Check sheet for the modelled part. Datum: model origin and axes. Units: mm. A direction names the side the tool comes from. Round coordinates to 2 decimals unless told otherwise and drop trailing zeros. Write each loop counter-clockwise with the first axis right and the second up, starting at its lowest first coordinate (ties: lowest second). Pieces come first, ordered by that corner, then holes.
Item 1: Cross-section at A-A on y = 0. Enter the section's corners in (x, z).
Item 2: Cross-section at C-C on x = 3.25. Enter the section's corners in (y, z).
Item 3: Cross-section at D-D on z = 1. Count the separate pieces of the cut face and the enclosed holes in it, plus the area to 3 significant figures.
Item 4: Cross-section at B-B on x = 1. Enter the section's corners in (y, z), plus the area to 3 significant figures.
Item 5: Go/stop test with flat-tipped pins: pin 1 Ø1.5 at (y, z) = (4.5, 5) entering from -X; pin 2 Ø1.4 at (x, y) = (-0.89, 3.33) entering from -Z; pin 3 Ø3 at (x, z) = (-3.5, 4) entering from +Y; pin 4 Ø3 at (y, z) = (4.5, 4) entering from +X. Record where each tip stops, or that it passes through.
Item 6: Material ranges on line 1 (Y direction, x = 1.25, z = 4); line 2 (Y direction, x = 0, z = 2.75); line 3 (X direction, y = -3.75, z = 3.5), recorded low to high.
Item 7: Tool access check on faces 4 (the flat face through (4.217, -3.502, 3.131)), 5 (the flat face through (-0.92, -5.4, 3.13)), 6 (the flat face through (-4.23, -3.46, 3.13)). Record the directions out of +Z, -Z, +X, -X, +Y, -Y that give a thin tool (end or side, any length) a straight path to the whole face; none if there is none.
Item 8: Release check for a two-part mould opening along Y. For faces 1 (the flat face through (-3.502, -4.217, 3.131)), 2 (the cylindrical face through (0, -2, 3)), 3 (the flat face through (-0.88, 5.39, 3.13)) record: +Y half, -Y half, draft (parallel to the pull), parting line (faces both ways), or undercut.
from build123d import *

# Parameters (mm, degrees)
SKETCH2_R           = 2
BOSS_EXTRUDE1_DEPTH = 6.35
SKETCH3_R           = 0.75
CUT_EXTRUDE1_DEPTH  = 11.490061241


with BuildPart() as part:
    # Sketch2 → Boss-Extrude1 (new body)
    with BuildSketch(Plane.XY):
        with BuildLine():
            Line((-5.904188549, -1.568559405), (-4.357072845, -2.241855531))
            ThreePointArc((-4.357072845, -2.241855531), (-4.248730253, -2.44096113), (-4.131295421, -2.634843097))
            Line((-4.131295421, -2.634843097), (-4.328897569, -4.310506566))
            Line((-4.328897569, -4.310506566), (-2.652408005, -4.120040264))
            ThreePointArc((-2.652408005, -4.120040264), (-2.459027768, -4.238299475), (-2.260385237, -4.347488767))
            Line((-2.260385237, -4.347488767), (-1.593681982, -5.897456974))
            Line((-1.593681982, -5.897456974), (-0.237032582, -4.894263536))
            ThreePointArc((-0.237032582, -4.894263536), (-0.010430778, -4.899988898), (0.216193347, -4.895228333))
            Line((0.216193347, -4.895228333), (1.568559405, -5.904188549))
            Line((1.568559405, -5.904188549), (2.241855531, -4.357072845))
            ThreePointArc((2.241855531, -4.357072845), (2.44096113, -4.248730253), (2.634843097, -4.131295421))
            Line((2.634843097, -4.131295421), (4.310506566, -4.328897569))
            Line((4.310506566, -4.328897569), (4.120040264, -2.652408005))
            ThreePointArc((4.120040264, -2.652408005), (4.238299475, -2.459027768), (4.347488767, -2.260385237))
            Line((4.347488767, -2.260385237), (5.897456974, -1.593681982))
            Line((5.897456974, -1.593681982), (4.894263536, -0.237032582))
            ThreePointArc((4.894263536, -0.237032582), (4.899988898, -0.010430778), (4.895228333, 0.216193347))
            Line((4.895228333, 0.216193347), (5.904188549, 1.568559405))
            Line((5.904188549, 1.568559405), (4.357072845, 2.241855531))
            ThreePointArc((4.357072845, 2.241855531), (4.248730253, 2.44096113), (4.131295421, 2.634843097))
            Line((4.131295421, 2.634843097), (4.328897569, 4.310506566))
            Line((4.328897569, 4.310506566), (2.652408005, 4.120040264))
            ThreePointArc((2.652408005, 4.120040264), (2.459027768, 4.238299475), (2.260385237, 4.347488767))
            Line((2.260385237, 4.347488767), (1.593681982, 5.897456974))
            Line((1.593681982, 5.897456974), (0.237032582, 4.894263536))
            ThreePointArc((0.237032582, 4.894263536), (0.010430778, 4.899988898), (-0.216193347, 4.895228333))
            Line((-0.216193347, 4.895228333), (-1.568559405, 5.904188549))
            Line((-1.568559405, 5.904188549), (-2.241855531, 4.357072845))
            ThreePointArc((-2.241855531, 4.357072845), (-2.44096113, 4.248730253), (-2.634843097, 4.131295421))
            Line((-2.634843097, 4.131295421), (-4.310506566, 4.328897569))
            Line((-4.310506566, 4.328897569), (-4.120040264, 2.652408005))
            ThreePointArc((-4.120040264, 2.652408005), (-4.238299475, 2.459027768), (-4.347488767, 2.260385237))
            Line((-4.347488767, 2.260385237), (-5.897456974, 1.593681982))
            Line((-5.897456974, 1.593681982), (-4.894263536, 0.237032582))
            ThreePointArc((-4.894263536, 0.237032582), (-4.899988898, 0.010430778), (-4.895228333, -0.216193347))
            Line((-4.895228333, -0.216193347), (-5.904188549, -1.568559405))
        make_face()
        Circle(SKETCH2_R, mode=Mode.SUBTRACT)
    extrude(amount=BOSS_EXTRUDE1_DEPTH)

    # Sketch3 → Cut-Extrude1 (cut, through all)
    with BuildSketch(Plane.XY.offset(6.35)):
        with Locations((-0.885829808, 3.334337348)):
            Circle(SKETCH3_R)
        with Locations((0.885829808, -3.334337348)):
            Circle(SKETCH3_R)
    extrude(amount=-CUT_EXTRUDE1_DEPTH, mode=Mode.SUBTRACT)


solid = part.part
Response values:
1. outline: (-4.9, 0) - (-2, 0) - (-2, 6.35) - (-4.9, 6.35) - close; (2, 0) - (4.9, 0) - (4.9, 6.35) - (2, 6.35) - close
2. outline: (-4.2, 0) - (4.19, 0) - (4.19, 6.35) - (-4.2, 6.35) - close
3. separate pieces: 1
3. enclosed holes: 3
3. area: 74.1 mm2
4. outline: (-5.48, 0) - (-4.08, 0) - (-4.08, 6.35) - (-5.48, 6.35) - close; (-2.59, 0) - (-1.73, 0) - (-1.73, 6.35) - (-2.59, 6.35) - close; (1.73, 0) - (5.46, 0) - (5.46, 6.35) - (1.73, 6.35) - close
4. area: 38.0 mm2
5. pin 1: stops at x = -4.31
5. pin 2: passes through
5. pin 3: stops at y = 4.91
5. pin 4: stops at x = 4.33
6. line 1: y = -5.67 to -3.99, -2.68 to -1.56, 1.56 to 5.64
6. line 2: y = -4.9 to -2, 2 to 4.9
6. line 3: x = -4.26 to 0.26, 1.51 to 4.24
7. face 4: +Z, -Z, +X
7. face 5: +Z, -Z, -Y
7. face 6: +Z, -Z, -X
8. face 1: -Y half
8. face 2: undercut
8. face 3: +Y half
